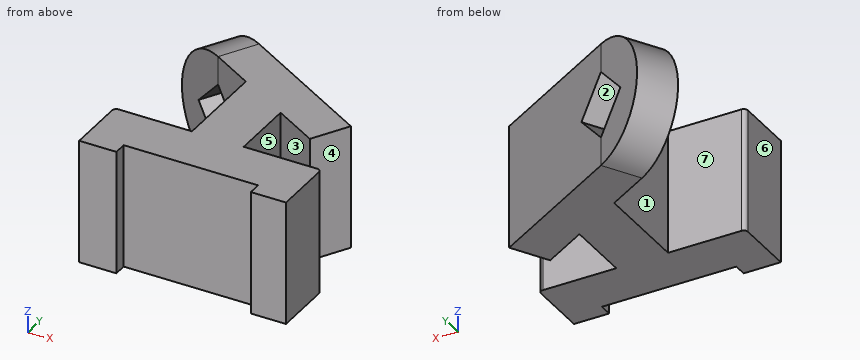
from build123d import *

# Parameters (mm, degrees)
BOSS_EXTRUDE1_DEPTH      = 38.1
BOSS_EXTRUDE1_DEPTH_BACK = 38.1
FILLET3_R                = 2.54
FILLET4_R                = 2.54
BOSS_EXTRUDE2_DEPTH      = 76.2
SKETCH6_R                = 38.1
BOSS_EXTRUDE3_DEPTH      = 25.4
CUT_EXTRUDE2_DEPTH       = 88.935283942


with BuildPart() as part:
    # Sketch1 → Boss-Extrude1 (new body, two sides)
    with BuildSketch(Plane.XY) as boss_extrude1_sk:
        Polygon((-78.057486297, 0), (-30.432486297, 0), (-30.432486297, 58.166), (1.317513703, 58.166), (1.317513703, 0), (48.942513703, 0), (48.942513703, -38.1), (27.352513703, -38.1), (27.352513703, -30.236305156), (-55.197486297, -30.236305156), (-55.197486297, -38.1), (-78.057486297, -38.1), align=None)
    extrude(amount=BOSS_EXTRUDE1_DEPTH)
    extrude(boss_extrude1_sk.sketch, amount=-BOSS_EXTRUDE1_DEPTH_BACK)

    # Fillet3
    fillet3_edges = [part.edges().sort_by_distance(p)[0] for p in [
        (48.942513703, 0, 0),
    ]]
    fillet(fillet3_edges, radius=FILLET3_R)

    # Fillet4
    fillet4_edges = [part.edges().sort_by_distance(p)[0] for p in [
        (-78.057486297, 0, 0),
    ]]
    fillet(fillet4_edges, radius=FILLET4_R)

    # Sketch5 → Boss-Extrude2 (add)
    with BuildSketch(Plane.XY.offset(38.1)):
        Polygon((-55.832486297, 72.830696837), (28.031248742, 24.411946837), (40.731248742, 46.408992094), (-43.132486297, 94.827742094), align=None)
    extrude(amount=-BOSS_EXTRUDE2_DEPTH)

    # Sketch6 → Boss-Extrude3 (add)
    with BuildSketch(Plane(origin=(30.278495244, 52.443892139, 0), x_dir=(0.866025404, -0.5, 0), z_dir=(0.5, 0.866025404, 0))):
        with Locations((-84.767699909, 0)):
            Circle(SKETCH6_R)
    extrude(amount=-BOSS_EXTRUDE3_DEPTH)

    # Sketch7 → Cut-Extrude2 (cut, through all)
    with BuildSketch(Plane(origin=(17.578495244, 30.446846883, 0), x_dir=(-0.866025404, 0.5, 0), z_dir=(-0.5, -0.866025404, 0))):
        Polygon((84.767699909, 20.574), (105.341699909, 0), (84.767699909, -20.574), (64.193699909, 0), align=None)
    extrude(amount=-CUT_EXTRUDE2_DEPTH, mode=Mode.SUBTRACT)


solid = part.part
Build history of the part. All positions in model axes, mm. Face numbers are marked on the shaded views. A direction names the side the tool comes from. Coordinates: 2 decimals unless noted, no trailing zeros. Order: outer loops, then holes, each group sorted by start corner. A loop starts at its lowest first (then second) coordinate and runs counter-clockwise, first axis right, second up. Notation, with made-up numbers: (40.25, 38.25) - (57.25, 38.25) arc R19 cw to (57.25, 60.25) - close; hole circle Ø1 at (84, 48.25). An arc over 180 degrees is marked (long way). Write item = value, one per line. Start each with the question number.
1) Saw through at D-D on z = 31. Write the cut outline in (x, y), then the cut area to 3 significant figures.
2) Saw through at B-B on x = 31. Write the cut outline in (y, z), then the cut area to 3 significant figures.
3) Two-plate mould, pull along X, no slides. Class the marked faces 5, 6 and 7: pulls with the +X half, pulls with the -X half, needs draft (parallel to the pull), parting line crosses it, or undercut.
4) 3-axis set-ups, long thin cutter, end or side, ignore diameter. For the marked faces 1, 2, 3 and 4: which of +Z, -Z, +X, -X, +Y, -Y reach the whole face in a straight line?
5) Saw through at C-C on y = 33.5. Write the cut outline in (x, z).
6) Flat gauge pins, fed straight in: pin 1 Ø1.5 at (y, z) = (40, -2.5) entering from -X; pin 2 Ø22.5 at (x, z) = (13.5, 12) entering from +Y; pin 3 Ø20 at (y, z) = (20.5, -11) entering from +X. Where does each tip first touch, or does it go through?
7) Wall check: line 1 along X through (y, z) = (-21, 33.5); line 2 along X through (y, z) = (26, 12); line 3 along X through (y, z) = (3, -14). Give the ranges that are in metal, low to high. Write a range as from..to.
8) Saw through at A-A on z = -2.5. Write the cut outline in (x, y), then the cut area to 3 significant figures.
From the geometry:
q1.outline = (-78.06, -38.1) - (-55.2, -38.1) - (-55.2, -30.24) - (27.35, -30.24) - (27.35, -38.1) - (48.94, -38.1) - (48.94, -2.54) arc R2.54 ccw to (46.4, 0) - (1.32, 0) - (1.32, 39.84) - (28.03, 24.41) - (40.73, 46.41) - (-62.31, 105.9) - (-75.01, 83.91) - (-30.43, 58.17) - (-30.43, 0) - (-75.52, 0) arc R2.54 ccw to (-78.06, -2.54) - close
q1.area = 8,760 mm^2
q2.outline = (-38.1, -38.1) - (0, -38.1) - (0, 38.1) - (-38.1, 38.1) - close; (29.55, -38.1) - (52.03, -38.1) - (52.03, 38.1) - (29.55, 38.1) - close
q2.area = 4,620 mm^2
q3.face_5 = undercut
q3.face_6 = pulls with the -X half
q3.face_7 = needs draft
q4.face_1 = +Z, -Z, -X
q4.face_2 = none
q4.face_3 = +Z, -Z
q4.face_4 = +Z, -Z, +X
q5.outline = (-30.43, -38.1) - (1.32, -38.1) - (1.32, 38.1) - (-30.43, 38.1) - close; (12.29, -38.1) - (33.28, -38.1) - (33.28, 38.1) - (12.29, 38.1) - close
q6.pin_1 = -30.43
q6.pin_2 = 68.63
q6.pin_3 = 31.55
q7.line_1 = -78.06..48.94
q7.line_2 = -30.43..1.32, 25.28..28.95
q7.line_3 = -30.43..1.32
q8.outline = (-88.76, 91.84) - (-71.49, 81.87) - (-58.79, 103.86) - (-76.06, 113.84) - close; (-78.06, -38.1) - (-55.2, -38.1) - (-55.2, -30.24) - (27.35, -30.24) - (27.35, -38.1) - (48.94, -38.1) - (48.94, -2.54) arc R2.54 ccw to (46.4, 0) - (1.32, 0) - (1.32, 39.84) - (28.03, 24.41) - (40.73, 46.41) - (-27.48, 85.79) - (-40.18, 63.79) - (-30.43, 58.17) - (-30.43, 0) - (-75.52, 0) arc R2.54 ccw to (-78.06, -2.54) - close
q8.area = 8,250 mm^2
